from build123d import *

# Parameters (mm, degrees)
F0_W     = 8.4666666667
F0_H     = 8.4666666667
F1_DEPTH = 0.127
F2_W     = 8.4666666667
F2_H     = 8.4666666667
F3_DEPTH = 0.254
F4_W     = 8.4666666667
F4_H     = 8.2126666667
F4_H_2   = 0.254
F5_DEPTH = 0.254


with BuildPart() as f1:
    # F0 (on Right) → F1 (new body, symmetric)
    with BuildSketch(Plane.YZ):
        Rectangle(F0_W, F0_H)
    extrude(amount=F1_DEPTH, both=True)

    # F2 (on face) → F3 (join)
    with BuildSketch(Plane(origin=(0, 0, -4.2333333333), x_dir=(1, 0, 0), z_dir=(0, 0, -1))):
        with Locations((4.3603333333, 0)):
            Rectangle(F2_W, F2_H)
    extrude(amount=-F3_DEPTH)

    # F4 (on face) → F5 (join)
    with BuildSketch(Plane.YZ.offset(8.5936666667)):
        with Locations((0, 0.127)):
            Rectangle(F4_W, F4_H)
        with Locations((0, -4.1063333333)):
            Rectangle(F4_W, F4_H_2)
    extrude(amount=F5_DEPTH)


solid = f1.part
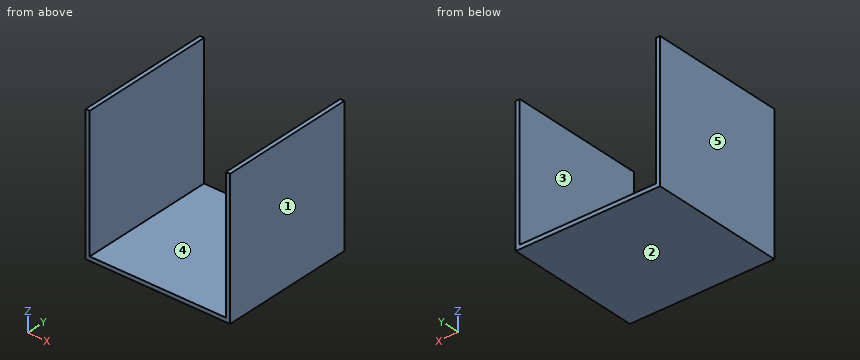
CAD build for the part. Positions are in the model's coordinates, mm. Face numbers are marked on the shaded views. A direction names the side the tool comes from. Round coordinates to 2 decimals unless told otherwise and drop trailing zeros. Loops run counter-clockwise (first coordinate to the right, second up) from the corner with the lowest first, then second, coordinate; pieces in that order, holes last. Notation, with made-up numbers: (-14, 38) - (34, 38) arc R16 ccw to (34, 65) - close; hole circle Ø4 at (31.25, -29.5). An arc over 180 degrees is marked (long way). Put each result on its own line as item: value.
1. Slice it at A-A on z = 2. List the corners of the cut face in (x, y).
Geometry check:
outline: (-0.13, -4.23) - (0.13, -4.23) - (0.13, 4.23) - (-0.13, 4.23) - close; (8.59, -4.23) - (8.85, -4.23) - (8.85, 4.23) - (8.59, 4.23) - close
2. Wall check: line 1 (X direction, y = 2.25, z = 2.5); line 2 (Z direction, x = 3.75, y = 2.5). Give the ranges that are in metal, low to high.
Geometry check:
line 1: -0.13 to 0.13, 8.59 to 8.85
line 2: -4.23 to -3.98
3. Slice it at C-C on x = 7. List the corners of the cut face in (y, z).
Geometry check:
outline: (-4.23, -4.23) - (4.23, -4.23) - (4.23, -3.98) - (-4.23, -3.98) - close
4. 3-axis set-ups, long thin cutter, end or side, ignore diameter. For the marked faces 4 and 5: which of +Z, -Z, +X, -X, +Y, -Y reach the whole face in a straight line?
Geometry check:
face 4: +Z, +Y, -Y
face 5: +Z, -Z, -X, +Y, -Y
5. Pin check, flat tip, straight feed: P1, Ø1, axis at x = 1.5, y = 2, coming from the +Z side. Stop position of the tip, or through.
Geometry check:
P1: z = -3.98
6. Slice it at B-B on y = 1.75. List the corners of the cut face in (x, z).
Geometry check:
outline: (-0.13, -4.23) - (8.85, -4.23) - (8.85, 4.23) - (8.59, 4.23) - (8.59, -3.98) - (0.13, -3.98) - (0.13, 4.23) - (-0.13, 4.23) - close
7. Two-plate mould, pull along X, no slides. Class the marked faces 1, 2 and 3: released by +X, released by -X, zero draft, split by the parting line, or undercut.
Geometry check:
face 1: released by +X
face 2: zero draft
face 3: undercut
